Could you check a few things on this model? Use its own coordinates, in mm. Face numbers are marked on the shaded views. A direction names the side the tool comes from. Coordinates: 2 decimals unless noted, no trailing zeros. Loops run counter-clockwise (first coordinate to the right, second up) from the corner with the lowest first, then second, coordinate; pieces in that order, holes last. Notation, with made-up numbers: (18, 68.5) -> (51, 68.5) arc R22 cw to (51, 79.5) -> close; hole circle Ø11 at (27, 83). An arc over 180 degrees is marked (long way). One line per question, with ' | ' between items.
from build123d import *

# Parameters (mm, degrees)
SALIENTE_EXTRUIR1_DEPTH = 24
CROQUIS3_R              = 1.55
CORTAR_EXTRUIR1_DEPTH   = 18.55
CORTAR_EXTRUIR2_DEPTH   = 17
CORTAR_EXTRUIR3_DEPTH   = 17


with BuildPart() as part:
    # Croquis2 → Saliente-Extruir1 (new body)
    with BuildSketch(Plane(origin=(0, 0, 0), x_dir=(1, 0, 0), z_dir=(0, 1, 0))):
        with BuildLine():
            Line((-7.55, 0), (-7.55, -7.55))
            Line((-7.55, -7.55), (-19.55, -7.55))
            Line((-19.55, -7.55), (-19.55, -4.55))
            Line((-19.55, -4.55), (-9.131754542, 4.075666691))
            ThreePointArc((-9.131754542, 4.075666691), (-2e-09, 10), (9.131754541, 4.075666695))
            Line((9.131754541, 4.075666695), (19.55, -4.55))
            Line((19.55, -4.55), (19.55, -7.55))
            Line((19.55, -7.55), (7.55, -7.55))
            Line((7.55, -7.55), (7.55, 0))
            ThreePointArc((7.55, 0), (0, 7.55), (-7.55, 0))
        make_face()
    extrude(amount=SALIENTE_EXTRUIR1_DEPTH)

    # Croquis3 → Cortar-Extruir1 (cut, through all)
    with BuildSketch(Plane.XY.offset(7.55)):
        with Locations((15, 12)):
            Circle(CROQUIS3_R)
        with Locations((-15, 12)):
            Circle(CROQUIS3_R)
    extrude(amount=-CORTAR_EXTRUIR1_DEPTH, mode=Mode.SUBTRACT)

    # Croquis4 → Cortar-Extruir2 (cut)
    with BuildSketch(Plane(origin=(0, 21, 0), x_dir=(1, 0, 0), z_dir=(0, 1, 0))):
        Polygon((-9.131754542, 4.075666691), (-19.55, -4.55), (-9.131754542, -4.55), align=None)
    extrude(amount=-CORTAR_EXTRUIR2_DEPTH, mode=Mode.SUBTRACT)

    # Croquis5 → Cortar-Extruir3 (cut)
    with BuildSketch(Plane(origin=(0, 21, 0), x_dir=(1, 0, 0), z_dir=(0, 1, 0))):
        Polygon((19.55, -4.55), (9.131754541, 4.075666695), (9.131754541, -4.55), align=None)
    extrude(amount=-CORTAR_EXTRUIR3_DEPTH, mode=Mode.SUBTRACT)


solid = part.part
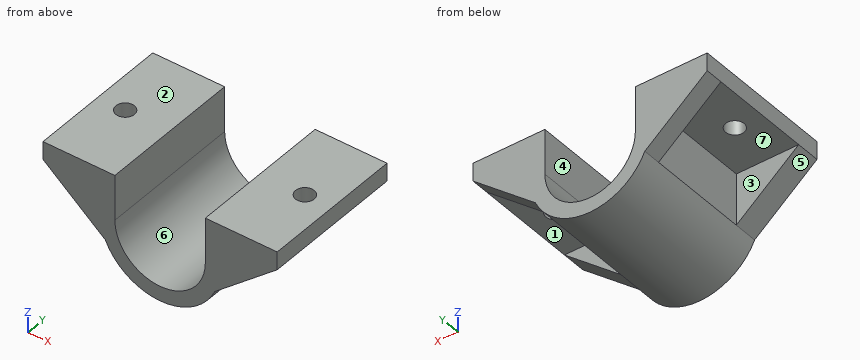
1) I'm going to push flat-ended pins straight in: pin 1 Ø8.5 at (x, y) = (17, 13.5) entering from -Z; pin 2 Ø4.5 at (y, z) = (11, 0.5) entering from -X; pin 3 Ø1 at (x, y) = (3.5, 20) entering from -Z; pin 4 Ø3 at (x, z) = (5, 2.5) entering from +Y. Where does each tip first touch, or does it pass through?
Data:
pin 1: z = 4.55 | pin 2: x = -9.13 | pin 3: z = -9.54 | pin 4: through
2) We'd pull the mould along X, two halves only. Please class the marked faces 5, 6 and 7: pulls with the +X half, pulls with the -X half, needs draft (parallel to the pull), parting line crosses it, or undercut.
Data:
face 5: pulls with the -X half | face 6: undercut | face 7: needs draft
3) If we section it at B-B on z = 3: Please give me the cut outline in (x, y), and give its area (3 significant figures).
Data:
outline: (-17.68, 0) -> (-7.55, 0) -> (-7.55, 24) -> (-17.68, 24) -> (-17.68, 21) -> (-9.13, 21) -> (-9.13, 4) -> (-17.68, 4) -> close; (7.55, 0) -> (17.68, 0) -> (17.68, 4) -> (9.13, 4) -> (9.13, 21) -> (17.68, 21) -> (17.68, 24) -> (7.55, 24) -> close | area: 196 mm²
4) I need wall thicknesses on line 1 along Y through (x, z) = (15, 6.05); line 2 along X through (y, z) = (6.75, 2); line 3 along Z through (x, y) = (10, 5.5). Which ranges of each line are inside material? Lowest first, please. Write a range as from..to.
Data:
line 1: 0..10.45, 13.55..24 | line 2: -9.13..-7.55, 7.55..9.13 | line 3: 4.55..7.55
5) If we section it at C-C on x = -15: Please give me the cut outline in (y, z).
Data:
outline: (0, 0.78) -> (4, 0.78) -> (4, 4.55) -> (10.45, 4.55) -> (10.45, 7.55) -> (0, 7.55) -> close; (13.55, 4.55) -> (21, 4.55) -> (21, 0.78) -> (24, 0.78) -> (24, 7.55) -> (13.55, 7.55) -> close
6) On a 3-axis mill with a long thin cutter (end or side, diameter ignored), from which of +Z, -Z, +X, -X, +Y, -Y can I reach the whole of each face in a straight line? I mean the marked faces 1, 2, 3 and 4. Say none if no direction works.
Data:
face 1: -Z, +X | face 2: +Z, +X, -X, +Y, -Y | face 3: -Z, -X | face 4: +Z, +Y, -Y
7) If we section it at A-A on y = 12: Please give me the cut outline in (x, z), and give its area (3 significant figures).
Data:
outline: (-19.55, 4.55) -> (-16.55, 4.55) -> (-16.55, 7.55) -> (-19.55, 7.55) -> close; (-13.45, 4.55) -> (-9.13, 4.55) -> (-9.13, -4.08) arc R10 ccw to (9.13, -4.08) -> (9.13, 4.55) -> (13.45, 4.55) -> (13.45, 7.55) -> (7.55, 7.55) -> (7.55, 0) arc R7.55 cw to (-7.55, 0) -> (-7.55, 7.55) -> (-13.45, 7.55) -> close; (16.55, 4.55) -> (19.55, 4.55) -> (19.55, 7.55) -> (16.55, 7.55) -> close | area: 131 mm²
8) If we section it at D-D on y = 7.25: Please give me the cut outline in (x, z), and give its area (3 significant figures).
Data:
outline: (-19.55, 4.55) -> (-9.13, 4.55) -> (-9.13, -4.08) arc R10 ccw to (9.13, -4.08) -> (9.13, 4.55) -> (19.55, 4.55) -> (19.55, 7.55) -> (7.55, 7.55) -> (7.55, 0) arc R7.55 cw to (-7.55, 0) -> (-7.55, 7.55) -> (-19.55, 7.55) -> close | area: 149 mm²
